Part print with two shaded views. Sizes in mm from the minimum x, y, z corner. A direction names the side the tool comes from. Coordinates: 2 decimals unless noted, no trailing zeros. Write each loop counter-clockwise with the first axis right and the second up, starting at its lowest first coordinate (ties: lowest second). Pieces come first, ordered by that corner, then holes. Notation, with made-up numbers: M 41.5,63 L 76.5,63 A23 ccw 76.5,98 Z; hole C 53.5,53 d9. An arc over 180 degrees is marked long. Use CSV: the item, a comma, the result in double quotes. Start each with the question number.
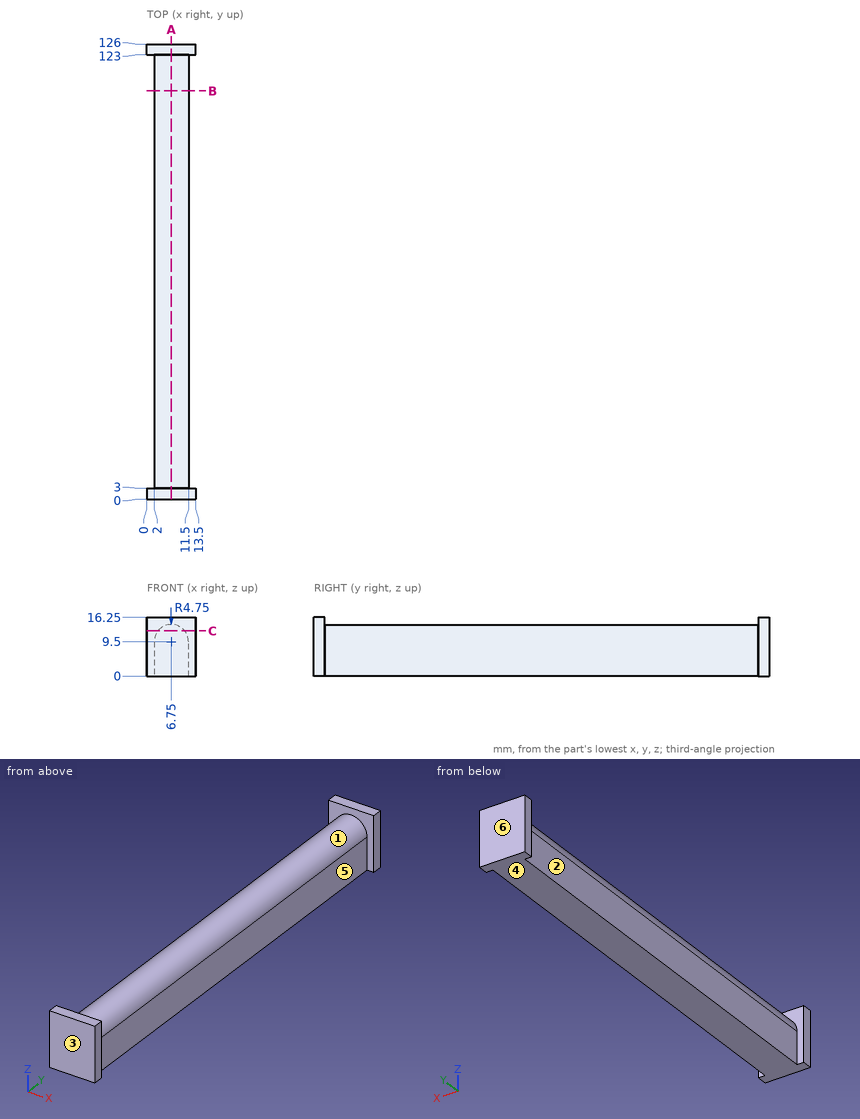
1. Pull direction Y, two halves, no side cores. Call the marked faces 3, 4, 5 and 6: pulls with the +Y half, pulls with the -Y half, needs draft (parallel to the pull), parting line crosses it, or undercut.
2. Slice it at A-A (x = 6.75). List the corners of the cut face in (y, z).
3. Flat gauge pins, fed straight in: pin 1 (4 mm diameter, centred on y = 63, z = 10, fed in from -X); pin 2 (1 mm diameter, centred on x = 3, y = 13, fed in from +Z); pin 3 (4 mm diameter, centred on x = 5.5, z = 7.5, fed in from -Y); pin 4 (6 mm diameter, centred on y = 17.5, z = 11, fed in from +X). Where does each tip first touch, or does it go through?
4. Slice it at C-C (z = 12.5). List the corners of the cut face in (x, y).
5. 3-axis set-ups, long thin cutter, end or side, ignore diameter. For the marked faces 1 and 2: which of +Z, -Z, +X, -X, +Y, -Y reach the whole face in a straight line?
6. Slice it at B-B (y = 113). List the corners of the cut face in (x, z), and give its area (3 significant figures).
7. Drill centre lines: line 1 along Y through (x, z) = (9.5, 14); line 2 along X through (y, z) = (58, 8.25); line 3 along Z through (x, y) = (3.5, 40.5). Where is each one in solid material? Low to high. Write a range as from..to.
Established:
1,face 3,"pulls with the -Y half"
1,face 4,"needs draft"
1,face 5,"undercut"
1,face 6,"pulls with the +Y half"
2,outline,"M 0,0 L 126,0 L 126,16.25 L 123,16.25 L 123,14.25 L 3,14.25 L 3,16.25 L 0,16.25 Z"
3,pin 1,"stops at x = 2"
3,pin 2,"stops at z = 12.96"
3,pin 3,"stops at y = 0"
3,pin 4,"stops at x = 11.5"
4,outline,"M 0,0 L 13.5,0 L 13.5,3 L 10.43,3 L 10.43,123 L 13.5,123 L 13.5,126 L 0,126 L 0,123 L 3.07,123 L 3.07,3 L 0,3 Z"
5,face 1,"+Z"
5,face 2,"+Z, -Z, -X"
6,outline,"M 2,0 L 11.5,0 L 11.5,9.5 A4.75 ccw 2,9.5 Z"
6,area,"126 mm2"
7,line 1,"y = 0..3, 123..126"
7,line 2,"x = 2..11.5"
7,line 3,"z = 0..12.96"
